Study the drawing (mm; zero at the part's minimum x, y, z) and answer. A direction names the side the tool comes from. Give positions to 0.01 mm unless a question says otherwise; leave off trailing zeros. Loops run counter-clockwise (first coordinate to the right, second up) from the corner with the lowest first, then second, coordinate; pieces in that order, holes last. Notation, with made-up numbers: (-27, 54.5) -> (-16, 54.5) arc R14 cw to (-16, 65.5) -> close; hole circle Ø2 at (64.5, 83). An arc over 180 degrees is marked (long way). One line per question, with ' | ' between items. Start each with the question number.
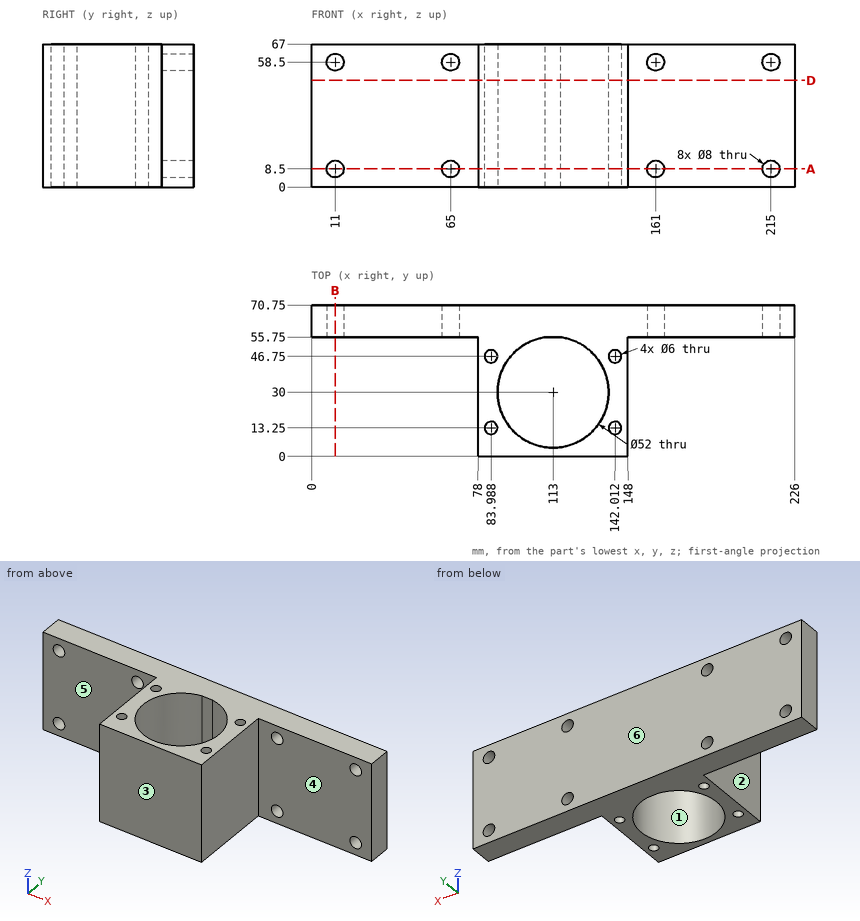
1. The part is cut by section B-B (x = 11). Write down the section's boundary in (y, z).
2. For the marked faces 4, 5 and 6, determine the directions among +Z, -Z, +X, -X, +Y, -Y from which every point of the face is accessible in a straight line to the end or side of a thin tool.
3. The part is cut by section D-D (z = 50). Write down the section's boundary in (x, y).
4. Straight lines are drawn through the part: L1, parallel to X at y = 65, z = 58; L2, parallel to Y at x = 150, z = 28.5; L3, parallel to Y at x = 111, z = 11.5. For each, find the intervals that lie inside material, in ascending order.
5. The part is cut by section A-A (z = 8.5). Count the separate pieces of the cut face and the enclosed holes in it, plus the area to 3 significant figures.
6. Determine the mould class of the marked faces 1, 2 and 3 for opening direction X: released by +X, released by -X, zero draft, split by the parting line, or undercut.
7. Each of these flat-tipped pins is pushed along its axis until it touches: pin 1 Ø8 at (y, z) = (32.5, 40) entering from -X; pin 2 Ø6 at (y, z) = (22.5, 11.5) entering from +X; pin 3 Ø5 at (x, z) = (183, 28.5) entering from -Y. Where does it stop, or does it pass through?
Check sheet entries:
1) outline: (55.75, 0) -> (70.75, 0) -> (70.75, 4.5) -> (55.75, 4.5) -> close; (55.75, 12.5) -> (70.75, 12.5) -> (70.75, 54.5) -> (55.75, 54.5) -> close; (55.75, 62.5) -> (70.75, 62.5) -> (70.75, 67) -> (55.75, 67) -> close
2) face 4: +Z, -Z, +X, -Y | face 5: +Z, -Z, -X, -Y | face 6: +Z, -Z, +X, -X, +Y
3) outline: (0, 55.75) -> (78, 55.75) -> (78, 0) -> (148, 0) -> (148, 55.75) -> (226, 55.75) -> (226, 70.75) -> (0, 70.75) -> close; hole circle Ø6 at (83.99, 13.25); hole circle Ø6 at (83.99, 46.75); hole (109.4, 55.75) arc R26 ccw (long way) to (116.6, 55.75) -> close; hole circle Ø6 at (142.01, 13.25); hole circle Ø6 at (142.01, 46.75)
4) L1: x = 0 to 7.03, 14.97 to 61.03, 68.97 to 157.03, 164.97 to 211.03, 218.97 to 226 | L2: y = 55.75 to 70.75 | L3: y = 0 to 4.08, 55.75 to 70.75
5) separate pieces: 5 | enclosed holes: 5 | area: 4,580 mm^2
6) face 1: undercut | face 2: released by -X | face 3: zero draft
7) pin 1: stops at x = 78 | pin 2: stops at x = 148 | pin 3: stops at y = 55.75
